The listing builds one solid part. Answer for the finished solid, in the listing's coordinates (mm). Coordinates: 2 decimals unless noted, no trailing zeros. Loops run counter-clockwise (first coordinate to the right, second up) from the corner with the lowest first, then second, coordinate; pieces in that order, holes last. Notation, with made-up numbers: M 24,81 L 57,81 A23 ccw 57,105 Z; hole C -2,-3.75 d7. An arc over 180 degrees is marked long. Answer as a JSON object with one key per item and string values. Group by question number.
1. Straight lines are drawn through the part: L1, parallel to Y at x = -3.5, z = 0; L2, parallel to Y at x = 7, z = 2; L3, parallel to Z at x = -11.5, y = 1. For each, find the intervals that lie inside material, in ascending order.
2. A cutting plane is placed at A-A on y = 0. Give the vertices of the cut face in (x, z), and give its area (3 significant figures).
3. A cutting plane is placed at C-C on x = -2.25. Give the vertices of the cut face in (y, z), and give its area (3 significant figures).
4. Given pin 1 (1 mm diameter, centred on x = -4, z = 3.5, fed in from -Y); pin 2 (3 mm diameter, centred on y = 0, z = 0, fed in from +X); pin 3 (3 mm diameter, centred on x = -4.5, y = 1.5, fed in from +Z); pin 4 (1 mm diameter, centred on x = 6, y = 2.5, fed in from +Z), each flat-ended and moving along its own axis, determine where each tip first touches the part or whether it passes through.
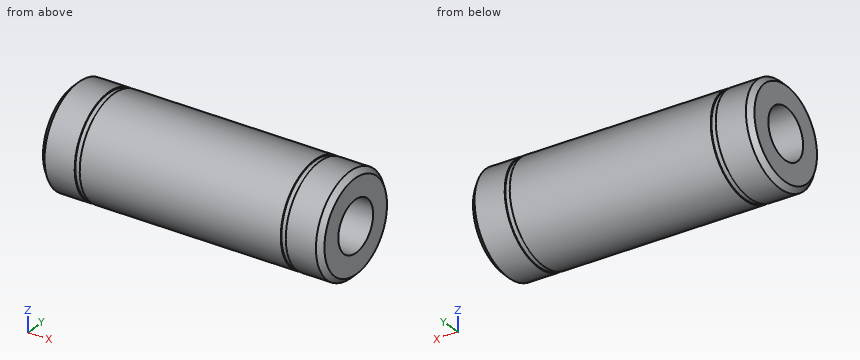
from build123d import *

# Parameters (mm, degrees)
SKETCH_1_R          = 5
SKETCH_1_R_2        = 2.5
EXTRUDE_1_DEPTH     = 14
CHAMFER_1_SIZE      = 0.5
CUT_EXTRUDE_START   = -10
SKETCH_3_OUTSIDE_W  = 18.274
SKETCH_3_OUTSIDE_H  = 18.274
SKETCH_3_OUTSIDE_R  = 4.9
CUT_EXTRUDE_1_DEPTH = 0.5


with BuildPart() as part:
    # 草图1 → 凸台-拉伸1 (new, symmetric)
    with BuildSketch(Plane(origin=(0, 0, 0), x_dir=(0, 0, -1), z_dir=(1, 0, 0))):
        Circle(SKETCH_1_R)
        Circle(SKETCH_1_R_2, mode=Mode.SUBTRACT)
    extrude(amount=EXTRUDE_1_DEPTH, both=True)

    # 倒角1
    chamfer_1_edges = [part.edges().sort_by_distance(p)[0] for p in [
        (-14, 0, 5),
        (14, 0, 5),
    ]]
    chamfer(chamfer_1_edges, length=CHAMFER_1_SIZE)

    # 草图3 outside → 切除-拉伸1 (cut)
    with BuildSketch(Plane(origin=(0, 0, 0), x_dir=(0, 0, -1), z_dir=(1, 0, 0)).offset(CUT_EXTRUDE_START)):
        Rectangle(SKETCH_3_OUTSIDE_W, SKETCH_3_OUTSIDE_H)
        Circle(SKETCH_3_OUTSIDE_R, mode=Mode.SUBTRACT)
    cut_extrude_1 = extrude(amount=-CUT_EXTRUDE_1_DEPTH, mode=Mode.SUBTRACT)

    # 镜向1: 切除-拉伸1 across plane
    add(cut_extrude_1.mirror(Plane(origin=(0, 0, 0), x_dir=(0, 0, 1), z_dir=(1, 0, 0))), mode=Mode.SUBTRACT)


solid = part.part
From the geometry:
{
 "1": {"L1": "y = -5 to -2.5, 2.5 to 5", "L2": "y = -4.58 to -1.5, 1.5 to 4.58", "L3": "z = -4.9 to -2.29, 2.29 to 4.9"},
 "2": {"outline": "M -14,-4.5 L -13.5,-5 L -10.5,-5 L -10.5,-4.9 L -10,-4.9 L -10,-5 L 10,-5 L 10,-4.9 L 10.5,-4.9 L 10.5,-5 L 13.5,-5 L 14,-4.5 L 14,-2.5 L -14,-2.5 Z; M -14,2.5 L 14,2.5 L 14,4.5 L 13.5,5 L 10.5,5 L 10.5,4.9 L 10,4.9 L 10,5 L -10,5 L -10,4.9 L -10.5,4.9 L -10.5,5 L -13.5,5 L -14,4.5 Z", "area": "139 mm²"},
 "3": {"outline": "C 0,0 d10; hole C 0,0 d5", "area": "58.9 mm²"},
 "4": {"pin 1": "stops at y = -4", "pin 2": "passes through", "pin 3": "stops at z = 5", "pin 4": "stops at z = 4.58"}
}
